Check sheet for the modelled part. Datum: model origin and axes. Units: mm. A direction names the side the tool comes from. Round coordinates to 2 decimals unless told otherwise and drop trailing zeros. Write each loop counter-clockwise with the first axis right and the second up, starting at its lowest first coordinate (ties: lowest second). Pieces come first, ordered by that corner, then holes. Notation, with made-up numbers: (-36, 38.5) -> (9, 38.5) arc R19 cw to (9, 44.5) -> close; hole circle Ø11 at (-10, 56.5). An arc over 180 degrees is marked (long way). Write item = value, one per line.
from build123d import *

# Parameters (mm, degrees)
SKETCH_1_W           = 48
SKETCH_1_H           = 18
EXTRUDE_1_DEPTH      = 3.5
SKETCH_6_W           = 18
SKETCH_6_H           = 9
EXTRUDE_4_DEPTH      = 25
SKETCH_7_R           = 3.5
CUT_EXTRUDE_1_DEPTH  = 2
SKETCH_9_R           = 5.5
CUT_EXTRUDE_4_DEPTH  = 3
EXTRUDE_5_OUTLINE_W  = 48
EXTRUDE_5_OUTLINE_H  = 18
EXTRUDE_5_DEPTH      = 20
CUT_EXTRUDE_7_REACH  = 98.344
SKETCH_13_R          = 3
SKETCH_13_R_2        = 1.25
SKETCH_15_R          = 6.7
CUT_EXTRUDE_8_DEPTH  = 45
SKETCH_16_R          = 3.15
CUT_EXTRUDE_9_DEPTH  = 76.081622399
EXTRUDE_6_REACH      = 56.196
SKETCH_17_W          = 18
SKETCH_17_H          = 3
SKETCH_18_W          = 14.545454545
SKETCH_18_H          = 18
EXTRUDE_7_DEPTH      = 2
SKETCH_19_W          = 22.545454545
SKETCH_19_H          = 18
CUT_EXTRUDE_11_DEPTH = 7
SKETCH_20_W          = 19.545454545
SKETCH_20_H          = 3
EXTRUDE_8_DEPTH      = 5
SKETCH_21_W          = 17
SKETCH_21_H          = 9
EXTRUDE_9_DEPTH      = 2
SKETCH_22_R          = 1.75
CUT_EXTRUDE_12_DEPTH = 73.152616166
SKETCH_24_W          = 3
SKETCH_24_H          = 18
CUT_EXTRUDE_13_DEPTH = 1
EXTRUDE_START        = 2
EXTRUDE_10_DEPTH     = 2


with BuildPart() as part:
    # 草圖1 → 填料-伸長1 (new, symmetric)
    with BuildSketch(Plane(origin=(0, 0, 0), x_dir=(1, 0, 0), z_dir=(0, 1, 0))):
        Rectangle(SKETCH_1_W, SKETCH_1_H)
    extrude(amount=EXTRUDE_1_DEPTH, both=True)

    # Sketch 3D_3 → Loft 1 section 0
    with BuildSketch(Plane(origin=(-44, 14.5, -9), x_dir=(0, -0.447213595499958, 0.894427190999916), z_dir=(-1, 0, 0))):
        with BuildLine():
            Line((0, 0), (16.099689438, 8.049844719))
            Line((16.099689438, 8.049844719), (20.124611797, 0))
            Line((20.124611797, 0), (4.024922359, -8.049844719))
            Line((4.024922359, -8.049844719), (0, 0))
        make_face()
    # 草圖5 → Loft 1 section 1
    with BuildSketch(Plane.ZY.offset(24)):
        with BuildLine():
            Line((-9, 3.5), (9, 3.5))
            Line((9, 3.5), (9, -3.5))
            Line((9, -3.5), (-9, -3.5))
            Line((-9, -3.5), (-9, 3.5))
        make_face()
    loft()

    # 草圖6 → 填料-伸長4 (add)
    with BuildSketch(Plane.ZY.offset(44)):
        with Locations((0, 10)):
            Rectangle(SKETCH_6_W, SKETCH_6_H)
    extrude(amount=EXTRUDE_4_DEPTH)

    # 草圖7 → 除料-伸長1 (cut)
    with BuildSketch(Plane.ZY.offset(69)):
        with Locations((0, 14.5)):
            Circle(SKETCH_7_R)
    extrude(amount=-CUT_EXTRUDE_1_DEPTH, mode=Mode.SUBTRACT)

    # Loft 1 2: read off the stored shape, not the designer's step
    # Loft 1 2: loft between two sections, ruled curve by curve
    loft_1_2_from = [
        Edge.make_bspline([(-67, 14.5, 3.5), (-67, 12.75, 3.5), (-67, 11, 2.333333333), (-67, 11, -2.333333333), (-67, 12.75, -3.5), (-67, 14.5, -3.5)], [0, 0, 0, 0, 0.5, 0.5, 1, 1, 1, 1], 3, [1, 0.666666667, 0.5, 0.5, 0.666666667, 1]),
        Edge.make_line((-67, 14.5, -3.5), (-67, 14.5, 3.5)),
    ]
    loft_1_2_to = [
        Edge.make_bspline([(-55, 15.833945938, 5.335783751), (-55, 12.063417219, 6.27841593), (-55, 9, 3.886572043), (-55, 9, -3.886572043), (-55, 12.063417219, -6.27841593), (-55, 15.833945938, -5.335783751)], [0, 0, 0, 0, 0.5, 0.5, 1, 1, 1, 1], 3, [1, 0.552953065, 0.4111804, 0.4111804, 0.552953065, 1]),
        Edge.make_line((-55, 15.833945938, -5.335783751), (-55, 15.833945938, 5.335783751)),
    ]
    loft_1_2 = Solid(Shell([*[Face.make_surface_from_curves(loft_1_2_from[k], loft_1_2_to[k]) for k in range(2)], Face(Wire(loft_1_2_from)), Face(Wire(loft_1_2_to))]))
    add(loft_1_2, mode=Mode.SUBTRACT)

    # 草圖9 → 除料-伸長4 (cut)
    with BuildSketch(Plane.ZY.offset(55)):
        with Locations((3.554e-06, 14.500000002)):
            Circle(SKETCH_9_R)
    extrude(amount=-CUT_EXTRUDE_4_DEPTH, mode=Mode.SUBTRACT)

    # 填料-伸長5: read off the stored shape, not the designer's step
    # 填料-伸長5 outline → 填料-伸長5 (add)
    with BuildSketch(Plane(origin=(0, 3.5, 0), x_dir=(1, 0, 0), z_dir=(0, 1, 0))):
        Rectangle(EXTRUDE_5_OUTLINE_W, EXTRUDE_5_OUTLINE_H)
    extrude(amount=EXTRUDE_5_DEPTH)

    # 草圖13 → 除料-伸長7 (cut, up to next)
    with BuildSketch(Plane.ZY.offset(-24), mode=Mode.PRIVATE) as cut_extrude_7_sk1:
        with Locations(Location((0, 14.5, 0), (0, 0, 180))):
            Circle(SKETCH_13_R)
    cut_extrude_7_tool1 = extrude(cut_extrude_7_sk1.sketch, amount=CUT_EXTRUDE_7_REACH, mode=Mode.PRIVATE) & part.part
    # 草圖13 → 除料-伸長7 (cut, up to next)
    with BuildSketch(Plane.ZY.offset(-24), mode=Mode.PRIVATE) as cut_extrude_7_sk2:
        with Locations(Location((-4.75, 14.5, 0), (0, 0, 180))):
            Circle(SKETCH_13_R_2)
    cut_extrude_7_tool2 = extrude(cut_extrude_7_sk2.sketch, amount=CUT_EXTRUDE_7_REACH, mode=Mode.PRIVATE) & part.part
    # 草圖13 → 除料-伸長7 (cut, up to next)
    with BuildSketch(Plane.ZY.offset(-24), mode=Mode.PRIVATE) as cut_extrude_7_sk3:
        with Locations(Location((4.75, 14.5, 0), (0, 0, 180))):
            Circle(SKETCH_13_R_2)
    cut_extrude_7_tool3 = extrude(cut_extrude_7_sk3.sketch, amount=CUT_EXTRUDE_7_REACH, mode=Mode.PRIVATE) & part.part
    add(cut_extrude_7_tool1.solids().sort_by_distance((24, 14.5, 0))[0], mode=Mode.SUBTRACT)
    add(cut_extrude_7_tool2.solids().sort_by_distance((24, 14.5, -4.75))[0], mode=Mode.SUBTRACT)
    add(cut_extrude_7_tool3.solids().sort_by_distance((24, 14.5, 4.75))[0], mode=Mode.SUBTRACT)

    # 草圖15 → 除料-伸長8 (cut)
    with BuildSketch(Plane(origin=(24, 0, 0), x_dir=(0, 0, -1), z_dir=(1, 0, 0))):
        with Locations((0, 14.5)):
            Circle(SKETCH_15_R)
    extrude(amount=-CUT_EXTRUDE_8_DEPTH, mode=Mode.SUBTRACT)

    # 草圖16 → 除料-伸長9 (cut, through all)
    with BuildSketch(Plane.XY.offset(9)):
        with Locations((15, 2.5)):
            Circle(SKETCH_16_R)
        with Locations((0, 2.5)):
            Circle(SKETCH_16_R)
        with Locations((-15, 2.5)):
            Circle(SKETCH_16_R)
    extrude(amount=-CUT_EXTRUDE_9_DEPTH, mode=Mode.SUBTRACT)

    # 填料-伸長6: up to this face of the body (flat: up to its plane)
    extrude_6_end = Plane(part.part.faces().sort_by_distance((-34, 9, 0))[0])
    # 草圖17 → 填料-伸長6 (add, up to the picked face)
    with BuildSketch(Plane.ZY.offset(24), mode=Mode.PRIVATE) as extrude_6_sk1:
        with Locations((0, 5)):
            Rectangle(SKETCH_17_W, SKETCH_17_H)
    extrude_6_tool1 = split(extrude(extrude_6_sk1.sketch, amount=EXTRUDE_6_REACH, mode=Mode.PRIVATE), bisect_by=extrude_6_end, keep=Keep.BOTH, mode=Mode.PRIVATE)
    add(extrude_6_tool1.solids().sort_by(Axis((-24, 5, 0), (-1, 0, 0)))[0])

    # 草圖18 → 填料-伸長7 (add)
    with BuildSketch(Plane.XZ.offset(-5.5)):
        with Locations((-36.727272728, 0)):
            Rectangle(SKETCH_18_W, SKETCH_18_H)
    extrude(amount=-EXTRUDE_7_DEPTH)

    # 草圖19 → 除料-伸長11 (cut)
    with BuildSketch(Plane(origin=(0, 7.5, 0), x_dir=(1, 0, 0), z_dir=(0, 1, 0))):
        with Locations((-40.727272728, 0)):
            Rectangle(SKETCH_19_W, SKETCH_19_H)
    extrude(amount=CUT_EXTRUDE_11_DEPTH, mode=Mode.SUBTRACT)

    # 草圖20 → 填料-伸長8 (add)
    with BuildSketch(Plane(origin=(0, 7.5, 0), x_dir=(1, 0, 0), z_dir=(0, 1, 0))):
        with Locations((-42.227272728, -7.5)):
            Rectangle(SKETCH_20_W, SKETCH_20_H)
    extrude_8 = extrude(amount=EXTRUDE_8_DEPTH)

    # 鏡射1: 填料-伸長8 across plane
    add(extrude_8.mirror(Plane.XY))

    # 草圖21 → 填料-伸長9 (add)
    with BuildSketch(Plane.XY.offset(9)):
        with Locations((-60.5, 10)):
            Rectangle(SKETCH_21_W, SKETCH_21_H)
    extrude_9 = extrude(amount=EXTRUDE_9_DEPTH)

    # 鏡射2: 填料-伸長9 across plane
    add(extrude_9.mirror(Plane.XY))

    # 草圖22 → 除料-伸長12 (cut, through all)
    with BuildSketch(Plane(origin=(0, 14.5, 0), x_dir=(1, 0, 0), z_dir=(0, 1, 0))):
        with Locations(Location((-62, -7.5, 0), (0, 0, 270))):
            Circle(SKETCH_22_R)
        with Locations(Location((-62, 7.5, 0), (0, 0, 270))):
            Circle(SKETCH_22_R)
    extrude(amount=-CUT_EXTRUDE_12_DEPTH, mode=Mode.SUBTRACT)

    # 草圖24 → 除料-伸長13 (cut)
    with BuildSketch(Plane(origin=(0, 7.5, 0), x_dir=(1, 0, 0), z_dir=(0, 1, 0))):
        with Locations((-30.954545455, 0)):
            Rectangle(SKETCH_24_W, SKETCH_24_H)
    extrude(amount=-CUT_EXTRUDE_13_DEPTH, mode=Mode.SUBTRACT)

    # 草圖25 → 填料-伸長10 (add)
    with BuildSketch(Plane.ZY.offset(69).offset(EXTRUDE_START)):
        with BuildLine():
            Line((3.5, 14.5), (11, 14.5))
            Line((11, 14.5), (11, 5.5))
            Line((11, 5.5), (-11, 5.5))
            Line((-11, 5.5), (-11, 14.5))
            Line((-11, 14.5), (-3.5, 14.5))
            ThreePointArc((-3.5, 14.5), (0, 11), (3.5, 14.5))
        make_face()
    extrude(amount=-EXTRUDE_10_DEPTH)


solid = part.part
(1) Material ranges on L1, parallel to X at y = 8, z = -7.5; L2, parallel to X at y = 6.75, z = 5.25; L3, parallel to X at y = 12.75, z = 7.5, recorded low to high. Write a range as [from, to].
Worked answers:
L1 = [-71, -63.75], [-60.25, -32.45], [-24, 24]
L2 = [-71, -32.45], [-24, 24]
L3 = [-71, -63.75], [-60.25, -52], [-24, 24]
(2) Sectioned sample at A-A on x = 15. Enter the section's corners in (y, z), then the cut area to 3 significant figures.
Worked answers:
outline = (-3.5, -9) -> (-0.65, -9) -> (-0.65, 9) -> (-3.5, 9) -> close; (5.65, -9) -> (23.5, -9) -> (23.5, 9) -> (5.65, 9) -> close; hole circle Ø13.4 at (14.5, 0)
area = 232 mm²
(3) Sectioned sample at B-B on x = 2. Enter the section's corners in (y, z), then the cut area to 3 significant figures.
Worked answers:
outline = (-3.5, -9) -> (0.07, -9) -> (0.07, 9) -> (-3.5, 9) -> close; (4.93, -9) -> (23.5, -9) -> (23.5, 9) -> (4.93, 9) -> close; hole circle Ø13.4 at (14.5, 0)
area = 257 mm²
(4) Access from +Z, -Z, +X, -X, +Y, -Y to the whole of each face (thin tool, end or side, straight path). Record for faces 1 (the flat face through (-58, 5.5, 0)), 2 (the flat face through (-42, 10, 6)), 3 (the flat face through (4, 10, -9)), 4 (the flat face through (-64, 14.5, -7)), 5 (the cylindrical face through (1.82, 7.96, 1.45)).
Worked answers:
face_1 = +Z, -Z, -X, -Y
face_2 = +Y
face_3 = -Z, +X, +Y, -Y
face_4 = +Z, -Z, -X, +Y
face_5 = +X
(5) Sectioned sample at C-C on x = -62. Count the separate pieces of the cut face and the enclosed holes in it, then the cut area to 3 significant figures.
Worked answers:
separate_pieces = 3
enclosed_holes = 0
area = 106 mm²
(6) Go/stop test with flat-tipped pins: P1, Ø1, axis at y = 18.5, z = -6, coming from the -X side; P2, Ø4, axis at x = -62, z = -7.5, coming from the +Y side; P3, Ø3, axis at x = 2, y = 7.5, coming from the -Z side; P4, Ø10, axis at x = -60.5, y = 0, coming from the -Z side. Record where each tip stops, or that it passes through.
Worked answers:
P1 = -24
P2 = 14.5
P3 = -9
P4 = through
(7) Release check for a two-part mould opening along Z. For faces 6 (the cylindrical face through (-63.55, 10.06, 8.31)), 7 (the flat face through (-42, 10, -9)), 8 (the cylindrical face through (-2.32, 4.63, 0.13)) record: pulls with the +Z half, pulls with the -Z half, needs draft (parallel to the pull), parting line crosses it, or undercut.
Worked answers:
face_6 = undercut
face_7 = pulls with the -Z half
face_8 = needs draft
